```python
from build123d import *

# Parameters (mm, degrees)
F2_W     = 0.8680555556
F2_H     = 1.6279645497
F3_DEPTH = 0.2
F4_COUNT = 4


# Not quite as in the source:
# - a feature names something its author has since deleted; it is built from what else it names


with BuildPart() as f1:
    # F0 (on Front) → F1 (revolve)
    with BuildSketch(Plane.XZ):
        with BuildLine():
            Line((0, 26.1458333333), (0, 0))
            Line((0, 0), (0.9097222222, 0))
            Line((0.9097222222, 0), (0.9097222222, 21.8055555556))
            ThreePointArc((0.9097222222, 21.8055555556), (0.6798471947, 24.0228515276), (0, 26.1458333333))
        make_face()
    revolve(axis=Axis((0, 0, 13.0729166667), (0, 0, 1)))

    # F2 (on Front) → F3 (join, symmetric)
    with BuildSketch(Plane.XZ):
        with Locations((0.4340277778, 0.8139822748)):
            Rectangle(F2_W, F2_H)
        with BuildLine():
            Line((0, 22.6730523746), (0, 1.6279645497))
            Line((0, 1.6279645497), (0.8680555556, 1.6279645497))
            Line((0.8680555556, 1.6279645497), (0.8680555556, 0))
            Line((0.8680555556, 0), (0.8680555556, -0.2430555556))
            Line((0.8680555556, -0.2430555556), (2.0138888889, -0.2430555556))
            Line((2.0138888889, -0.2430555556), (2.0138888889, 0.5902777778))
            Line((2.0138888889, 0.5902777778), (3.0902777778, 0.5902777778))
            Line((3.0902777778, 0.5902777778), (2.6215277778, 2.3958333333))
            Line((2.6215277778, 2.3958333333), (0.8, 2.3958333333))
            Line((0.8, 2.3958333333), (0.8, 2.6680555556))
            Line((0.8, 2.6680555556), (1.1180555556, 2.9861111111))
            Line((1.1180555556, 2.9861111111), (1.1180555556, 3.2638888889))
            Line((1.1180555556, 3.2638888889), (2.0138888889, 3.2638888889))
            Line((2.0138888889, 3.2638888889), (2.0138888889, 13.3944219874))
            ThreePointArc((2.0138888889, 13.3944219874), (1.7758643131, 14.3441874312), (1.1180555556, 15.0694444444))
            Line((1.1180555556, 15.0694444444), (1.1180555556, 19.6012199821))
            Line((1.1180555556, 19.6012199821), (0, 22.6730523746))
        make_face()
    extrude(amount=F3_DEPTH, both=True)

    # F4: F1 ×4 about axis
    f4_axis = Axis((0, 0, 0), (0, 0, 1))


with BuildPart() as f1_1:
    add(f1.part)
    for i in range(1, F4_COUNT):
        add(f1.part.rotate(f4_axis, i * 360 / F4_COUNT))


solid = f1_1.part
```
Could you check a few things on this model? Use its own coordinates, in mm. A direction names the side the tool comes from. Give positions to 0.01 mm unless a question says otherwise; leave off trailing zeros. Loops run counter-clockwise (first coordinate to the right, second up) from the corner with the lowest first, then second, coordinate; pieces in that order, holes last. Notation, with made-up numbers: (80, 12) - (92, 12) arc R24 ccw to (92, 46) - close; hole circle Ø8 at (5.5, -23). An arc over 180 degrees is marked (long way). Answer in a Markdown table with one row per item. Add a question column.
Q1. If we section it at D-D (z = 14): List the corners of the cut face in (x, y) for me.
Q2. Which directions (+Z, -Z, +X, -X, +Y, -Y) give clear straight access to the entire face, cutting with the end or side of a thin tool? Please do faces 1 (the face through (1.8, 0, 14.3)), 2 (the face through (-1.4, -0.2, 9.7)), 3 (the face through (0.2, -1.4, 9.7)), 4 (the face through (1.4, 0.2, 9.7)), 5 (the face through (-0.2, 1.4, 9.7)).
Q3. For pin 1 (1.1 mm diameter, centred on x = -2.5, z = 1.5, fed in from -Y); pin 2 (2.5 mm diameter, centred on x = 2.5, z = 1.5, fed in from +Y); pin 3 (3 mm diameter, centred on y = -1.5, z = 20.5, fed in from +X), each with a flat end and sliding along its axis, tell me the tip position at first contact or that it passes through.
Q4. If we section it at B-B (z = 17.5): List the corners of the cut face in (x, y) for me.
Q5. Please list where these lines run through material, in increasing order: L1, parallel to Y at x = -1.5, z = 14.5; L2, parallel to Y at x = -0.25, z = 17. Write a range as from..to.
Q6. If we section it at A-A (x = 1.75): List the corners of the cut face in (y, z) for me, plus the area to 3 significant figures.
The answers:
| question | item | result |
|---|---|---|
| 1 | outline | (-1.92, -0.2) - (-0.89, -0.2) arc R0.91 ccw to (-0.2, -0.89) - (-0.2, -1.92) - (0.2, -1.92) - (0.2, -0.89) arc R0.91 ccw to (0.89, -0.2) - (1.92, -0.2) - (1.92, 0.2) - (0.89, 0.2) arc R0.91 ccw to (0.2, 0.89) - (0.2, 1.92) - (-0.2, 1.92) - (-0.2, 0.89) arc R0.91 ccw to (-0.89, 0.2) - (-1.92, 0.2) - close |
| 2 | face 1 | +Z, +X, +Y, -Y |
| 2 | face 2 | +Z, -Z, -X, -Y |
| 2 | face 3 | +Z, -Z, +X, -Y |
| 2 | face 4 | +Z, -Z, +X, +Y |
| 2 | face 5 | +Z, -Z, -X, +Y |
| 3 | pin 1 | stops at y = -0.2 |
| 3 | pin 2 | stops at y = 0.2 |
| 3 | pin 3 | stops at x = 1.06 |
| 4 | outline | (-1.12, -0.2) - (-0.89, -0.2) arc R0.91 ccw to (-0.2, -0.89) - (-0.2, -1.12) - (0.2, -1.12) - (0.2, -0.89) arc R0.91 ccw to (0.89, -0.2) - (1.12, -0.2) - (1.12, 0.2) - (0.89, 0.2) arc R0.91 ccw to (0.2, 0.89) - (0.2, 1.12) - (-0.2, 1.12) - (-0.2, 0.89) arc R0.91 ccw to (-0.89, 0.2) - (-1.12, 0.2) - close |
| 5 | L1 | y = -0.2..0.2 |
| 5 | L2 | y = -0.87..0.87 |
| 6 | outline | (-0.2, -0.24) - (0.2, -0.24) - (0.2, 2.4) - (-0.2, 2.4) - close; (-0.2, 3.26) - (0.2, 3.26) - (0.2, 14.39) - (-0.2, 14.39) - close |
| 6 | area | 5.51 mm^2 |
